Design review of the part built by this model. Coordinates are the model's own, in mm. A direction names the side the tool comes from. Round coordinates to 2 decimals unless told otherwise and drop trailing zeros. Order: outer loops, then holes, each group sorted by start corner. A loop starts at its lowest first (then second) coordinate and runs counter-clockwise, first axis right, second up. Notation, with made-up numbers: (72, 6) - (86, 6) arc R32 cw to (86, 44) - close; hole circle Ø9 at (49.25, 38.25). An arc over 180 degrees is marked (long way). Answer as a JSON object with one key per item and string values. Group by question number.
from build123d import *

# Parameters (mm, degrees)
SKETCH1_W           = 10
SKETCH1_H           = 10
BOSS_EXTRUDE1_DEPTH = 85
SKETCH2_W           = 10
SKETCH2_H           = 15
CUT_EXTRUDE1_DEPTH  = 4
SKETCH3_R           = 10.75
BOSS_EXTRUDE2_DEPTH = 3
SKETCH4_R           = 1
CUT_EXTRUDE2_DEPTH  = 3
SKETCH5_R           = 1.5
CUT_EXTRUDE3_DEPTH  = 1


with BuildPart() as part:
    # Sketch1 → Boss-Extrude1 (new body, symmetric)
    with BuildSketch(Plane(origin=(0, 0, 0), x_dir=(1, 0, 0), z_dir=(0, 1, 0))):
        Rectangle(SKETCH1_W, SKETCH1_H)
    extrude(amount=BOSS_EXTRUDE1_DEPTH, both=True)

    # Sketch2 → Cut-Extrude1 (cut)
    with BuildSketch(Plane.XY.offset(5)):
        Rectangle(SKETCH2_W, SKETCH2_H)
    extrude(amount=-CUT_EXTRUDE1_DEPTH, mode=Mode.SUBTRACT)

    # Sketch3 → Boss-Extrude2 (add)
    with BuildSketch(Plane.XZ.offset(85)):
        Circle(SKETCH3_R)
    extrude(amount=BOSS_EXTRUDE2_DEPTH)

    # Sketch4 → Cut-Extrude2 (cut)
    with BuildSketch(Plane(origin=(0, -85, 0), x_dir=(1, 0, 0), z_dir=(0, 1, 0))):
        with Locations((8, 0)):
            Circle(SKETCH4_R)
        with Locations((0, -8)):
            Circle(SKETCH4_R)
        with Locations((-8, 0)):
            Circle(SKETCH4_R)
        with Locations((0, 8)):
            Circle(SKETCH4_R)
    extrude(amount=-CUT_EXTRUDE2_DEPTH, mode=Mode.SUBTRACT)

    # Sketch5 → Cut-Extrude3 (cut)
    with BuildSketch(Plane(origin=(0, -85, 0), x_dir=(1, 0, 0), z_dir=(0, 1, 0))):
        with Locations((8, 0)):
            Circle(SKETCH5_R)
        with Locations((0, -8)):
            Circle(SKETCH5_R)
        with Locations((-8, 0)):
            Circle(SKETCH5_R)
        with Locations((0, 8)):
            Circle(SKETCH5_R)
    extrude(amount=-CUT_EXTRUDE3_DEPTH, mode=Mode.SUBTRACT)


solid = part.part
1. Clearance check with flat-ended pins moving along their axes: P1, Ø0.9, axis at x = 7.5, z = 0.5, coming from the +Y side; P2, Ø11, axis at x = 2.5, y = 19, coming from the -Z side; P3, Ø3.5, axis at x = -0.5, z = 8, coming from the +Y side. State where each tip first meets the part, or that it passes through.
2. Take a section at A-A, the plane z = 3.25. Give the boundary of the cut face in (x, y).
3. Take a section at B-B, the plane y = -29. Give the boundary of the cut face in (x, z).
4. Mouldability with a two-part tool opening along Y and no side actions: class faces 1 (the flat face through (0, 85, 0)), 2 (the flat face through (0, -7.5, 3)), 3 (the cylindrical face through (-1.4, -86.48, 10.66)) as pulls with the +Y half, pulls with the -Y half, needs draft (parallel to the pull), parting line crosses it, or undercut.
5. Take a section at C-C, the plane y = 4.5. Give the boundary of the cut face in (x, z).
6. Tool access review of faces 4 (the cylindrical face through (-9.5, -85.49, -0.07)), 5 (the flat face through (0, 1, -5)), 6 (the flat face through (0, 7.5, 3)), 7 (the flat face through (0, -46, 5)): name each direction out of +Z, -Z, +X, -X, +Y, -Y from which nothing blocks a thin tool from reaching the whole face with its end or side.
7. To check wall thickness, follow line 1 (Y direction, x = -9.5, z = -1.75); line 2 (Z direction, x = -2.25, y = 9.5). State the ranges of each line that lie inside material, in increasing order. Write a range as from..to.
Response values:
{
 "1": {"P1": "y = -86", "P2": "z = -5", "P3": "y = -85"},
 "2": {"outline": "(-10.25, -88) - (10.25, -88) - (10.25, -85) - (5, -85) - (5, -7.5) - (-5, -7.5) - (-5, -85) - (-10.25, -85) - close; (-5, 7.5) - (5, 7.5) - (5, 85) - (-5, 85) - close"},
 "3": {"outline": "(-5, -5) - (5, -5) - (5, 5) - (-5, 5) - close"},
 "4": {"face 1": "pulls with the +Y half", "face 2": "undercut", "face 3": "needs draft"},
 "5": {"outline": "(-5, -5) - (5, -5) - (5, 1) - (-5, 1) - close"},
 "6": {"face 4": "+Y", "face 5": "-Z, +X, -X, +Y", "face 6": "+Z, +X, -X", "face 7": "+Z, +X, -X, +Y"},
 "7": {"line 1": "-88..-85", "line 2": "-5..5"}
}
